Here's how the part is built. I have some questions about the finished solid (model axes, mm). A direction names the side the tool comes from. Give positions to 0.01 mm unless a question says otherwise; leave off trailing zeros. Loops run counter-clockwise (first coordinate to the right, second up) from the corner with the lowest first, then second, coordinate; pieces in that order, holes last. Notation, with made-up numbers: M 8,-24.5 L 32,-24.5 A19 ccw 32,-3.5 Z; hole C 83,67.25 d7. An arc over 180 degrees is marked long. Answer as CSV lines item,"result". Start each with the question number.
Item 1: I want a section at A-A on y = -1. List the corners of the cut face in (x, z) for me.
Item 2: I want a section at C-C on x = 31. List the corners of the cut face in (y, z) for me, plus the area to 3 significant figures.
Item 3: Will this pin go through, and if not, where does the flat tip stop? P1, Ø3, axis at y = -4, z = -45, coming from the -X side.
Item 4: I want a section at B-B on z = -24.5. List the corners of the cut face in (x, y) for me, plus the area to 3 significant figures.
Item 5: If I drill on line 1 along Y through (x, z) = (33.5, -33); line 2 along X through (y, z) = (-0.5, -15.5); line 3 along X through (y, z) = (-0.75, -46), over which ranges is the centre line in solid material (lowest first)? Write a range as from..to.
Item 6: For faces 1 (the flat face through (20, -5, -47)), 2 (the cylindrical face through (18.175, -1.479, -18.131)), which set-ups out of +Z, -Z, +X, -X, +Y, -Y let a thin tool reach every point of the face, with its end or its side?
from build123d import *

# Parameters (mm, degrees)
SALIENTE_EXTRUIR1_DEPTH = 2
REDONDEO1_R             = 2
CROQUIS4_R              = 3
SALIENTE_EXTRUIR2_DEPTH = 7
REDONDEO2_R             = 2


with BuildPart() as part:
    # Croquis1 → Saliente-Extruir1 (new body)
    with BuildSketch(Plane(origin=(0, 0, 0), x_dir=(1, 0, 0), z_dir=(0, 1, 0))):
        Polygon((63, 0), (69, 0), (78, 18), (78, 45), (69, 63), (63, 63), (0, 63), (0, 0), align=None)
    extrude(amount=SALIENTE_EXTRUIR1_DEPTH)

    # Redondeo1
    redondeo1_edges = [part.edges().sort_by_distance(p)[0] for p in [
        (0, 1, -63),
        (0, 1, 0),
    ]]
    fillet(redondeo1_edges, radius=REDONDEO1_R)

    # Croquis4 → Saliente-Extruir2 (add)
    with BuildSketch(Plane(origin=(0, 2, 0), x_dir=(1, 0, 0), z_dir=(0, 1, 0))):
        with Locations(Location((20, 47.25, 0), (0, 0, 270))):
            Circle(CROQUIS4_R)
        with Locations(Location((20, 15.75, 0), (0, 0, 270))):
            Circle(CROQUIS4_R)
        with Locations(Location((58, 31.5, 0), (0, 0, 270))):
            Circle(CROQUIS4_R)
    extrude(amount=-SALIENTE_EXTRUIR2_DEPTH)

    # Redondeo2
    redondeo2_edges = [part.edges().sort_by_distance(p)[0] for p in [
        (20, -5, -50.25),
        (20, -5, -18.75),
        (58, -5, -34.5),
    ]]
    fillet(redondeo2_edges, radius=REDONDEO2_R)


solid = part.part
Result:
1,outline,"C 20,-47.25 d6; C 20,-15.75 d6; C 58,-31.5 d6"
2,outline,"M 0,-63 L 2,-63 L 2,0 L 0,0 Z"
2,area,"126 mm^2"
3,P1,"x = 17.17"
4,outline,"M 0,0 L 78,0 L 78,2 L 0,2 Z"
4,area,"156 mm^2"
5,line 1,"0..2"
5,line 2,"17.01..22.99"
5,line 3,"17.27..22.73"
6,face 1,"+Z, -Z, +X, -X, -Y"
6,face 2,"-Y"
